```python
from build123d import *

# Parameters (mm, degrees)
BOSS_EXTRUDE1_DEPTH = 2
BOSS_EXTRUDE2_DEPTH = 3.2
CUT_EXTRUDE1_DEPTH  = 4.200000092
FILLET1_R           = 10


with BuildPart() as part:
    # Sketch3 → Boss-Extrude1 (new body)
    with BuildSketch(Plane.XY.offset(13)):
        Polygon((-3.57e-07, 1.6), (8.295592088, 1.6), (8.93017926, 1.6), (8.934835346, -1.6), (8.268122338, -1.6), (-8.285812718, -1.6), (-8.869806966, -1.6), (-8.865150879, 1.6), (-8.277696583, 1.6), align=None)
    extrude(amount=-BOSS_EXTRUDE1_DEPTH)

    # Sketch4 → Boss-Extrude2 (add)
    with BuildSketch(Plane.XZ.offset(1.6)):
        Polygon((-7.949410938, 13.000000268), (7.949410938, 13.000000268), (7.949410938, 13.080862351), (5.549410824, 14.200000092), (-5.549410824, 14.200000092), (-7.949410938, 13.080862351), align=None)
    extrude(amount=-BOSS_EXTRUDE2_DEPTH)

    # Sketch5 → Cut-Extrude1 (cut, through all)
    with BuildSketch(Plane(origin=(0, 0, 11), x_dir=(-1, 0, 0), z_dir=(0, 0, -1))):
        with BuildLine():
            ThreePointArc((-0.03251419, -1.6), (-4.481346725, -1.006559792), (-8.93017926, -1.6))
            Line((-8.93017926, -1.6), (-0.03251419, -1.6))
        make_face()
        with BuildLine():
            ThreePointArc((8.865150879, -1.6), (4.416318345, -1.006559792), (-0.03251419, -1.6))
            Line((-0.03251419, -1.6), (8.865150879, -1.6))
        make_face()
        with BuildLine():
            Line((8.865150879, 1.6), (-0.03251419, 1.6))
            ThreePointArc((-0.03251419, 1.6), (4.416318345, 1.006559792), (8.865150879, 1.6))
        make_face()
        with BuildLine():
            Line((-0.03251419, 1.6), (-8.93017926, 1.6))
            ThreePointArc((-8.93017926, 1.6), (-4.481346725, 1.006559792), (-0.03251419, 1.6))
        make_face()
    extrude(amount=-CUT_EXTRUDE1_DEPTH, mode=Mode.SUBTRACT)

    # Fillet1
    fillet1_edges = [part.edges().sort_by_distance(p)[0] for p in [
        (0.03251419, -1.6, 12.600000046),
        (0.03251419, 1.6, 12.600000046),
    ]]
    fillet(fillet1_edges, radius=FILLET1_R)


solid = part.part
```
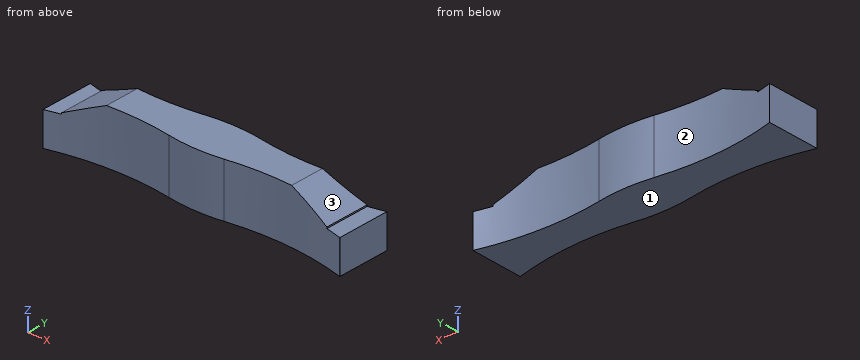
Model file for the job. Use its own axes, mm. Face numbers are marked on the shaded views. Coordinates: 2 decimals unless noted, no trailing zeros. Loops run counter-clockwise (first coordinate to the right, second up) from the corner with the lowest first, then second, coordinate; pieces in that order, holes last. Notation, with made-up numbers: (71.5, 32.25) - (121.5, 32.25) arc R16 cw to (121.5, 47.25) - close; hole circle Ø1 at (31.25, 81). An arc over 180 degrees is marked (long way). Answer as a JSON object with one key per item and string values. Group by question number.
(1) Probe line 1 along X through (y, z) = (-0.35, 11.65); line 2 along X through (y, z) = (0.55, 13.05); line 3 along Y through (x, z) = (-5.5, 13.6). List the from-to ranges inside material, lowest first.
(2) Flat gauge pin, fed straight in: pin 1 (0.7 mm diameter, centred on x = -8.5, y = 0.5, fed in from +Z). Where does the tip first touch, or does it go through?
(3) Cut at D-D (x = 3.25). Give the cut face in (y, z), then the cut area to 3 significant figures.
(4) Two-plate mould, pull along X, no slides. Class the marked faces 1, 2 and 3: released by +X, released by -X, zero draft, split by the parting line, or undercut.
(5) Cut at B-B (x = -5). Give the cut face in (y, z).
(6) Cut at A-A (y = -0.85). Give the cut face in (x, z), then the cut area to 3 significant figures.
Geometry says:
{
 "1": {"line 1": "x = -8.87 to 8.93", "line 2": "x = -7.95 to 7.95", "line 3": "y = -1.04 to 1.04"},
 "2": {"pin 1": "stops at z = 13"},
 "3": {"outline": "(-1.05, 11) - (1.05, 11) - (1.05, 14.2) - (-1.05, 14.2) - close", "area": "6.73 mm^2"},
 "4": {"face 1": "zero draft", "face 2": "undercut", "face 3": "released by +X"},
 "5": {"outline": "(-1.02, 11) - (1.02, 11) - (1.02, 14.2) - (-1.02, 14.2) - close"},
 "6": {"outline": "(-8.87, 11) - (8.93, 11) - (8.93, 13) - (7.95, 13) - (7.95, 13.08) - (5.55, 14.2) - (-5.55, 14.2) - (-7.95, 13.08) - (-7.95, 13) - (-8.87, 13) - close", "area": "52.0 mm^2"}
}
